Source: CAD feature listing. Evaluate the final solid. Frame: model axes, mm. A direction names the side the tool comes from. Coordinates: 2 decimals unless noted, no trailing zeros. Order: outer loops, then holes, each group sorted by start corner. A loop starts at its lowest first (then second) coordinate and runs counter-clockwise, first axis right, second up. Notation, with made-up numbers: (42, -9) -> (52, -9) arc R23 ccw to (52, 7) -> close; hole circle Ø8 at (0.5, -30.5). An arc over 180 degrees is marked (long way). Write each question's results on one line, items separated by ' | '. Start each with the question number.
Solid Edge part; units mm, degrees
sketch "Sketch1" plane through (0, 0, 0) normal (0, 0, 1) x (1, 0, 0)
  line L0 (-16, -7.9) -> (16, -7.9)
  line L1 (16, -7.9) -> (16, 7.9)
  line L2 (16, 7.9) -> (-16, 7.9)
  line L3 (-16, 7.9) -> (-16, -7.9)
  dimension "D1" = 16
extrude "Protrusion1" add sketch "Sketch1" along normal blind 3.1
sketch "Sketch2" plane through (0, 0, 0) normal (0, 0, -1) x (1, 0, 0)
  line L0 (-14.45, -6.45) -> (14.45, -6.45)
  line L1 (14.45, -6.45) -> (14.45, 6.45)
  line L2 (14.45, 6.45) -> (-14.45, 6.45)
  line L3 (-14.45, 6.45) -> (-14.45, -6.45)
extrude "ExtrudedCutout_2" cut sketch "Sketch2" against normal blind 1.8
sketch "Sketch3" plane through (0, 0, 3.1) normal (0, 0, 1) x (1, 0, 0)
  circle A0 centre (-4, 4) radius 2.4
  circle A1 centre (4, 4) radius 2.4
  circle A2 centre (12, 4) radius 2.4
  circle A3 centre (12, -4) radius 2.4
  circle A4 centre (4, -4) radius 2.4
  circle A5 centre (-4, -4) radius 2.4
  circle A6 centre (-12, -4) radius 2.4
  circle A7 centre (-12, 4) radius 2.4
  dimension "D1" = 12
extrude "ExtrudedProtrusion_4" add sketch "Sketch3" along normal blind 1.8
sketch "Sketch4" plane through (0, 0, 0) normal (0, 0, -1) x (-1, 0, 0)
  circle A0 centre (12, 4) radius 1.5
  circle A1 centre (12, -4) radius 1.5
  circle A2 centre (4, -4) radius 1.5
  circle A3 centre (4, 4) radius 1.5
  circle A4 centre (-4, 4) radius 1.5
  circle A5 centre (-4, -4) radius 1.5
  circle A6 centre (-12, -4) radius 1.5
  circle A7 centre (-12, 4) radius 1.5
extrude "ExtrudedCutout_4" cut sketch "Sketch4" against normal blind 4.8
sketch "Sketch5" plane through (0, 0, 1.8) normal (0, 0, -1) x (-1, 0, 0)
  circle A0 centre (-8, 0) radius 3.2
  circle A1 centre (0, 0) radius 3.2
  circle A2 centre (8, 0) radius 3.2
  circle A3 centre (8, 0) radius 2.4
  circle A4 centre (0, 0) radius 2.4
  circle A5 centre (-8, 0) radius 2.4
extrude "Protrusion2" add sketch "Sketch5" along normal blind 1.8
sketch "Sketch6" plane through (0, -7.9, 1.55) normal (0, -1, 0) x (1, 0, 0)
  line L0 (-16, -1.55) -> (-16, 1.55)
  line L1 (-16, 1.55) -> (16, 1.55)
  line L2 (16, 1.55) -> (16, -1.55)
  line L3 (16, -1.55) -> (-16, -1.55)
extrude "ExtrudedProtrusion_9" add sketch "Sketch6" along normal blind 0.1
sketch "Sketch7" plane through (0, 7.9, 1.55) normal (0, 1, 0) x (-1, 0, 0)
  line L0 (-16, -1.55) -> (-16, 1.55)
  line L1 (-16, 1.55) -> (16, 1.55)
  line L2 (16, 1.55) -> (16, -1.55)
  line L3 (16, -1.55) -> (-16, -1.55)
extrude "Protrusion3" add sketch "Sketch7" along normal blind 0.1
(1) Section D-D on x = -4. Return the cut outline in (y, z), then the cut area to 3 significant figures.
(2) Section C-C on z = 2.5. Count the separate pieces of the cut face and the enclosed holes in it, then the cut area to 3 significant figures.
(3) Section A-A on z = 0.55. Return the cut outline in (x, y).
(4) Draft query along X for faces 1 (the cylindrical face through (10.398, -0.106, 0.913)), 2 (the flat face through (0, -8, 2)), 3 (the flat face through (16, 0, 2)). Return one class per face: released by +X, released by -X, zero draft, split by the parting line, or undercut.
(5) Reachability of faces 4 (the flat face through (0, 7, 0)), 5 (the cylindrical face through (2.57, 4.45, 3.28)), 6 (the cylindrical face through (-14.398, 3.894, 3.987)) from +Z, -Z, +X, -X, +Y, -Y: full face, straight path, thin tool, end or side. Return the list, or none.
(6) Line query: L1, parallel to Y at x = -8, z = 0.4; L2, parallel to Y at x = -4, z = 4.25; L3, parallel to Y at x = -12, z = 2.45. Output: solid intervals per line, ascending.
(7) First-contact query: P1, Ø1, axis at x = 11, z = 4, coming from the +Y side; P2, Ø1.5, axis at x = 4, y = -4, coming from the -Z side; P3, Ø3.5, axis at x = 4.5, y = 4.5, coming from the -Z side. Flat tips, straight axial feed; report the tip coordinate or a pass-through.
Results list:
1) outline: (-8, 0) -> (-6.45, 0) -> (-6.45, 1.8) -> (-5.5, 1.8) -> (-5.5, 4.8) -> (-2.5, 4.8) -> (-2.5, 1.8) -> (2.5, 1.8) -> (2.5, 4.8) -> (5.5, 4.8) -> (5.5, 1.8) -> (6.45, 1.8) -> (6.45, 0) -> (8, 0) -> (8, 3.1) -> (6.4, 3.1) -> (6.4, 4.9) -> (1.6, 4.9) -> (1.6, 3.1) -> (-1.6, 3.1) -> (-1.6, 4.9) -> (-6.4, 4.9) -> (-6.4, 3.1) -> (-8, 3.1) -> close | area: 25.7 mm²
2) separate pieces: 1 | enclosed holes: 8 | area: 455 mm²
3) outline: (-16, -8) -> (16, -8) -> (16, 8) -> (-16, 8) -> close; circle Ø6.4 at (-8, 0); circle Ø6.4 at (0, 0); circle Ø6.4 at (8, 0); hole (-14.45, -6.45) -> (14.45, -6.45) -> (14.45, 6.45) -> (-14.45, 6.45) -> close; hole circle Ø4.8 at (-8, 0); hole circle Ø4.8 at (0, 0); hole circle Ø4.8 at (8, 0)
4) face 1: undercut | face 2: zero draft | face 3: released by +X
5) face 4: -Z, +X, -X, +Y, -Y | face 5: -Z | face 6: +Z
6) L1: y = -8 to -6.45, -3.2 to -2.4, 2.4 to 3.2, 6.45 to 8 | L2: y = -6.4 to -5.5, -2.5 to -1.6, 1.6 to 2.5, 5.5 to 6.4 | L3: y = -8 to -5.5, -2.5 to 2.5, 5.5 to 8
7) P1: stops at y = 6.35 | P2: stops at z = 4.8 | P3: stops at z = 1.8
